Input: part model. Units: mm. Frame: model coordinates. A direction names the side the tool comes from. Give positions to 0.01 mm unless a question says otherwise; leave off trailing zeros. Write each loop counter-clockwise with the first axis right and the second up, starting at its lowest first coordinate (ties: lowest second). Pieces come first, ordered by that corner, then holes. Notation, with made-up numbers: (51, 85.5) - (64, 85.5) arc R7 cw to (64, 97.5) - close; hole circle Ø10 at (-21, 38). An arc over 180 degrees is marked (long way). Answer as CSV lines item,"result". Start each with the question number.
from build123d import *

# Parameters (mm, degrees)
SKETCH1_W           = 290
SKETCH1_H           = 175
BOSS_EXTRUDE1_DEPTH = 140
SKETCH2_W           = 25.4
SKETCH2_H           = 175
BOSS_EXTRUDE2_DEPTH = 98.8
SKETCH3_W           = 25
SKETCH3_H           = 11.396117448
BOSS_EXTRUDE3_DEPTH = 100


with BuildPart() as part:
    # Sketch1 → Boss-Extrude1 (new body)
    with BuildSketch(Plane(origin=(0, 0, 0), x_dir=(1, 0, 0), z_dir=(0, 1, 0))):
        Rectangle(SKETCH1_W, SKETCH1_H)
    extrude(amount=BOSS_EXTRUDE1_DEPTH)

    # Sketch2 → Boss-Extrude2 (add)
    with BuildSketch(Plane.XZ):
        with Locations((87.7, 0)):
            Rectangle(SKETCH2_W, SKETCH2_H)
    extrude(amount=BOSS_EXTRUDE2_DEPTH)

    # Sketch3 → Boss-Extrude3 (add)
    with BuildSketch(Plane(origin=(145, 0, 0), x_dir=(0, 0, -1), z_dir=(1, 0, 0))):
        with Locations((0, 36.066217011)):
            Rectangle(SKETCH3_W, SKETCH3_H)
    extrude(amount=BOSS_EXTRUDE3_DEPTH)


solid = part.part
1) Cut plane B-B on x = 17. Output: boundary loops of the cut face in (y, z), and give its area (3 significant figures).
2) Reachability of faces 4 (the flat face through (194, 36, -12.5)), 5 (the flat face through (-37, 0, -1)), 6 (the flat face through (194, 41.764, 0)), 7 (the flat face through (122, 0, -1)), 8 (the flat face through (194, 36, 12.5)) from +Z, -Z, +X, -X, +Y, -Y: full face, straight path, thin tool, end or side. Return the list, or none.
3) Cut plane A-A on z = 58.5. Output: boundary loops of the cut face in (x, y).
4) Pull-direction query (X, two-part tool) for faces 1 (the flat face through (-2, 72, 87.5)), 2 (the flat face through (75, -49, -1)), 3 (the flat face through (245, 36, 0)); classes: +X half, -X half, draft (parallel to the pull), parting line (faces both ways), or undercut.
5) Contact query for flat-ended pins moving along their axis: P1, Ø3.5, axis at x = 219, y = 36.5, coming from the -Z side; P2, Ø3, axis at x = 107, z = 57, coming from the -Y side; P3, Ø5.5, axis at x = 210.5, y = 38.5, coming from the +Z side. Output: stop coordinate, or through.
6) Material intervals for line 1 (Y direction, x = -83, z = 38); line 2 (X direction, y = -60.5, z = -75.5); line 3 (X direction, y = 105, z = 70.5), sorted ascending. Write a range as from..to.
7) Cut plane C-C on y = 91.5. Output: boundary loops of the cut face in (x, z), and give its area (4 significant figures).
Numbers:
1,outline,"(0, -87.5) - (140, -87.5) - (140, 87.5) - (0, 87.5) - close"
1,area,"24,500 mm²"
2,face 4,"-Z, +X, +Y, -Y"
2,face 5,"+Z, -Z, -X, -Y"
2,face 6,"+Z, -Z, +X, +Y"
2,face 7,"+Z, -Z, +X, -Y"
2,face 8,"+Z, +X, +Y, -Y"
3,outline,"(-145, 0) - (75, 0) - (75, -98.8) - (100.4, -98.8) - (100.4, 0) - (145, 0) - (145, 140) - (-145, 140) - close"
4,face 1,"draft"
4,face 2,"-X half"
4,face 3,"+X half"
5,P1,"stops at z = -12.5"
5,P2,"stops at y = 0"
5,P3,"stops at z = 12.5"
6,line 1,"y = 0..140"
6,line 2,"x = 75..100.4"
6,line 3,"x = -145..145"
7,outline,"(-145, -87.5) - (145, -87.5) - (145, 87.5) - (-145, 87.5) - close"
7,area,"50,750 mm²"
